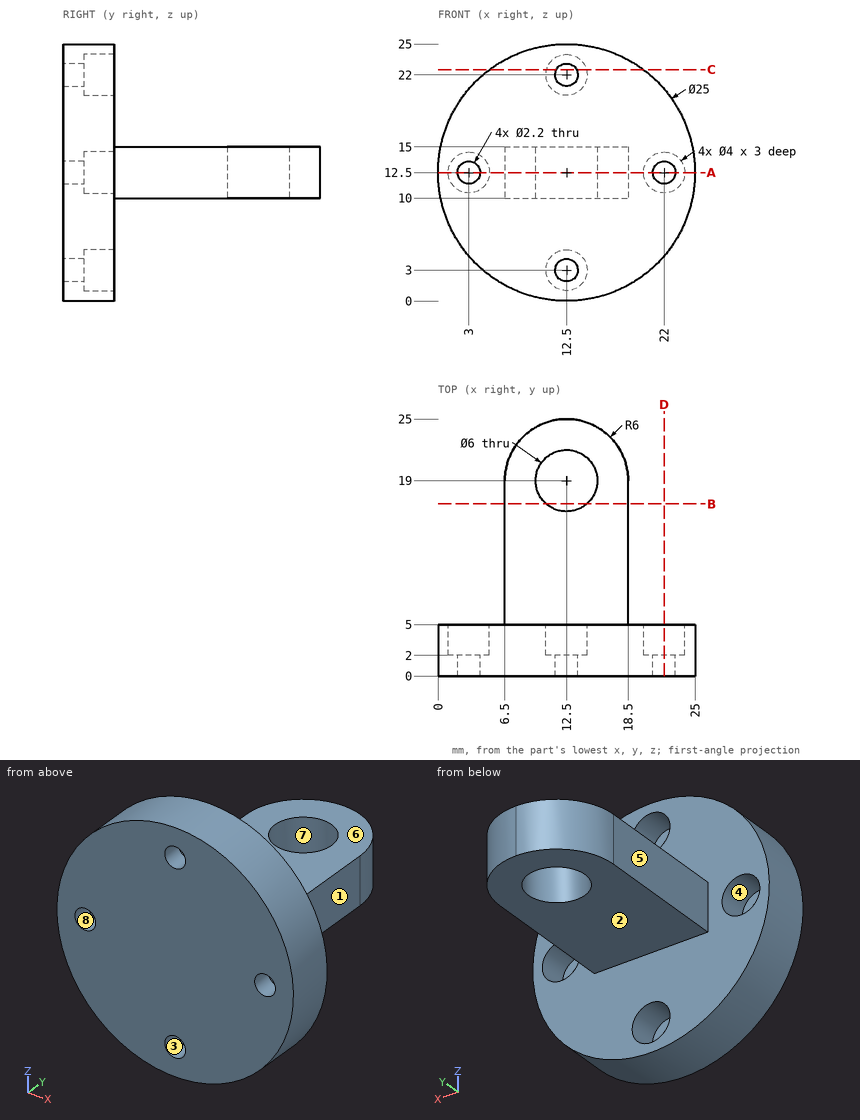
Job drawing, mm, ordinate dimensions from the low corner. One solid piece. A direction names the side the tool comes from. Round coordinates to 2 decimals unless told otherwise and drop trailing zeros. Write each loop counter-clockwise with the first axis right and the second up, starting at its lowest first coordinate (ties: lowest second). Pieces come first, ordered by that corner, then holes. Notation, with made-up numbers: (-6.5, 59.25) -> (51.5, 59.25) arc R29 cw to (51.5, 93.25) -> close; hole circle Ø1 at (28, 33.25). An arc over 180 degrees is marked (long way). Answer as a JSON object with one key per item and string values.
(1) Two-plate mould, pull along Z, no slides. Class the marked faces 1, 2 and 3: +Z half, -Z half, draft (parallel to the pull), parting line (faces both ways), or undercut.
Reported:
{"face 1": "draft", "face 2": "-Z half", "face 3": "undercut"}
(2) Which spindle directions (+Z, -Z, +X, -X, +Y, -Y) get a long thin tool onto all of the face, cutting with end or side? Do the marked faces 4, 5, 6, 7 and 8. Say none if no direction does.
Reported:
{"face 4": "+Y", "face 5": "+Z, -Z, -X, +Y", "face 6": "+Z, +X, -X, +Y", "face 7": "+Z, -Z", "face 8": "+Y, -Y"}
(3) Band-saw the part on C-C, the plane z = 22.5. List the corners of the cut face in (x, y), then the cut area to 3 significant figures.
Reported:
{"outline": "(5, 0) -> (11.52, 0) -> (11.52, 2) -> (10.56, 2) -> (10.56, 5) -> (5, 5) -> close; (13.48, 0) -> (20, 0) -> (20, 5) -> (14.44, 5) -> (14.44, 2) -> (13.48, 2) -> close", "area": "59.5 mm^2"}
(4) Pin check, flat tips, straight feed: P1, Ø1.8, axis at x = 3, z = 12.5, coming from the -Y side; P2, Ø1.2, axis at x = 21.5, z = 13, coming from the +Y side; P3, Ø10, axis at x = 5, y = 18, coming from the +Z side; P4, Ø10, axis at x = 9.5, y = 9.5, coming from the +Z side. Stop position of each tip, or through.
Reported:
{"P1": "passes through", "P2": "stops at y = 2", "P3": "stops at z = 15", "P4": "stops at z = 24.97"}
(5) Band-saw the part on A-A, the plane z = 12.5. List the corners of the cut face in (x, y), then the cut area to 3 significant figures.
Reported:
{"outline": "(0, 0) -> (1.9, 0) -> (1.9, 2) -> (1, 2) -> (1, 5) -> (0, 5) -> close; (4.1, 0) -> (20.9, 0) -> (20.9, 2) -> (20, 2) -> (20, 5) -> (18.5, 5) -> (18.5, 19) arc R6 ccw to (6.5, 19) -> (6.5, 5) -> (5, 5) -> (5, 2) -> (4.1, 2) -> close; (23.1, 0) -> (25, 0) -> (25, 5) -> (24, 5) -> (24, 2) -> (23.1, 2) -> close; hole circle Ø6 at (12.5, 19)", "area": "288 mm^2"}
(6) Probe probe 1 along X at (y, z) = (3.3, 12.5); probe 2 along X at (y, z) = (1.4, 12.5); probe 3 along Z at (x, y) = (12.75, 4.5). List the from-to ranges inside material, lowest first. Write a range as [from, to].
Reported:
{"probe 1": "x = [0, 1], [5, 20], [24, 25]", "probe 2": "x = [0, 1.9], [4.1, 20.9], [23.1, 25]", "probe 3": "z = [0, 1.02], [4.98, 20.02], [23.98, 25]"}
(7) Band-saw the part on B-B, the plane y = 16.75. List the corners of the cut face in (x, z).
Reported:
{"outline": "(6.5, 10) -> (10.52, 10) -> (10.52, 15) -> (6.5, 15) -> close; (14.48, 10) -> (18.5, 10) -> (18.5, 15) -> (14.48, 15) -> close"}
(8) Band-saw the part on D-D, the plane x = 22. List the corners of the cut face in (y, z).
Reported:
{"outline": "(0, 4.38) -> (5, 4.38) -> (5, 10.5) -> (2, 10.5) -> (2, 11.4) -> (0, 11.4) -> close; (0, 13.6) -> (2, 13.6) -> (2, 14.5) -> (5, 14.5) -> (5, 20.62) -> (0, 20.62) -> close"}
